from build123d import *
from OCP.BRepFilletAPI import BRepFilletAPI_MakeChamfer

# Parameters (mm, degrees)
SKETCH1_R           = 10
BOSS_EXTRUDE1_DEPTH = 28.5
BOSS_EXTRUDE2_DEPTH = 45
CUT_EXTRUDE1_DEPTH  = 30
CIRPATTERN1_COUNT   = 2
CHAMFER1_SIZE       = 50
CHAMFER1_SIZE2      = 13.397459622
FILLET3_R           = 15
CHAMFER2_SIZE       = 90
CHAMFER2_SIZE2      = 13.607292824
CUT_EXTRUDE2_DEPTH  = 138.877715566
CUT_EXTRUDE4_DEPTH  = 22.15
FILLET6_R           = 6.35


with BuildPart() as part:
    # Sketch1 → Boss-Extrude1 (new body)
    with BuildSketch(Plane.XY):
        Polygon((-9.192766332, -123.5075), (41.607233668, 123.5075), (9.192766332, 123.5075), (-41.607233668, -123.5075), align=None)
        with Locations(Location((0, 0, 0), (0, 0, 180))):
            Circle(SKETCH1_R, mode=Mode.SUBTRACT)
    extrude(amount=BOSS_EXTRUDE1_DEPTH)

    # Sketch2 → Boss-Extrude2 (add)
    with BuildSketch(Plane(origin=(0, 0, 0), x_dir=(-1, 0, 0), z_dir=(0, 0, -1))):
        Polygon((-41.607233668, 123.5075), (-38.473043437, 108.2675), (-6.0585761, 108.2675), (-9.192766332, 123.5075), align=None)
        Polygon((38.473043437, -108.2675), (6.0585761, -108.2675), (9.192766332, -123.5075), (41.607233668, -123.5075), align=None)
    extrude(amount=BOSS_EXTRUDE2_DEPTH)

    # Sketch4 → Cut-Extrude1 (cut)
    with BuildSketch(Plane(origin=(0, 123.5075, 0), x_dir=(1, 0, 0), z_dir=(0, 1, 0))):
        with BuildLine():
            ThreePointArc((20.6375, 30.433032299), (22.032403955, 27.065436254), (25.4, 25.670532299))
            Line((25.4, 25.670532299), (25.4, 30.433032299))
            Line((25.4, 30.433032299), (20.6375, 30.433032299))
        make_face()
        with BuildLine():
            Line((25.4, 30.433032299), (25.4, 25.670532299))
            ThreePointArc((25.4, 25.670532299), (28.767596045, 27.065436254), (30.1625, 30.433032299))
            Line((30.1625, 30.433032299), (25.4, 30.433032299))
        make_face()
        with BuildLine():
            Line((20.6375, 30.433032299), (25.4, 30.433032299))
            Line((25.4, 30.433032299), (25.4, 35.195532299))
            ThreePointArc((25.4, 35.195532299), (22.032403955, 33.800628344), (20.6375, 30.433032299))
        make_face()
        with BuildLine():
            Line((25.4, 35.195532299), (25.4, 30.433032299))
            Line((25.4, 30.433032299), (30.1625, 30.433032299))
            ThreePointArc((30.1625, 30.433032299), (28.767596045, 33.800628344), (25.4, 35.195532299))
        make_face()
    cut_extrude1 = extrude(amount=-CUT_EXTRUDE1_DEPTH, mode=Mode.SUBTRACT)

    # CirPattern1: Cut-Extrude1 ×2 about axis
    cirpattern1_axis = Axis((0, 0, 28.5), (0, 0, -1))
    for i in range(1, CIRPATTERN1_COUNT):
        add(cut_extrude1.rotate(cirpattern1_axis, i * 360 / CIRPATTERN1_COUNT), mode=Mode.SUBTRACT)

    # Chamfer1: one chamfer whose edges measure the first distance from different faces: ONE call of the kernel's chamfer builder (chamfer() names one face for all edges)
    chamfer1_edges_1 = [part.edges().sort_by_distance(p)[0] for p in [
        (-25.4, -123.5075, 28.5),
    ]]
    chamfer1_side_1 = [part.faces().sort_by_distance(p)[0] for p in [
        (-25.4, -123.5075, -7.566085514),
    ]]
    chamfer1_edges_2 = [part.edges().sort_by_distance(p)[0] for p in [
        (25.4, 123.5075, 28.5),
    ]]
    chamfer1_side_2 = [part.faces().sort_by_distance(p)[0] for p in [
        (25.4, 123.5075, -7.566085514),
    ]]
    chamfer1 = BRepFilletAPI_MakeChamfer(part.part.solid().wrapped)
    for e in chamfer1_edges_1:
        chamfer1.Add(CHAMFER1_SIZE, CHAMFER1_SIZE2, e.wrapped, chamfer1_side_1[0].wrapped)  # the first distance lies on this face
    for e in chamfer1_edges_2:
        chamfer1.Add(CHAMFER1_SIZE, CHAMFER1_SIZE2, e.wrapped, chamfer1_side_2[0].wrapped)  # the first distance lies on this face
    add(Compound.cast(chamfer1.Shape()), mode=Mode.REPLACE)

    # Fillet3
    fillet3_edges = [part.edges().sort_by_distance(p)[0] for p in [
        (22.265809769, 108.2675, 0),
        (-22.265809769, -108.2675, 0),
    ]]
    fillet(fillet3_edges, radius=FILLET3_R)

    # Chamfer2
    chamfer2_edges = [part.edges().sort_by_distance(p)[0] for p in [
        (-22.644738381, -110.110040378, 28.5),
        (22.644738381, 110.110040378, 28.5),
    ]]
    chamfer2_side = [part.faces().sort_by_distance(p)[0] for p in [
        (13.919836124, 0.470415947, 28.5),
    ]]
    chamfer(chamfer2_edges, length=CHAMFER2_SIZE, length2=CHAMFER2_SIZE2, reference=chamfer2_side[0])

    # Sketch10 → Cut-Extrude2 (cut, symmetric)
    with BuildSketch(Plane(origin=(0, 0, 0), x_dir=(0, 0, -1), z_dir=(1, 0, 0))):
        with BuildLine():
            Line((-28.5, 20.110040378), (-11.939027322, 98.927851264))
            ThreePointArc((-11.939027322, 98.927851264), (-4.989688501, 112.1926981), (7.875417438, 119.856804105))
            Line((7.875417438, 119.856804105), (-24.698068362, 128.387749722))
            Line((-24.698068362, 128.387749722), (-33.956814005, 23.522391457))
            Line((-33.956814005, 23.522391457), (-28.5, 20.110040378))
        make_face()
    cut_extrude2 = extrude(amount=CUT_EXTRUDE2_DEPTH, both=True, mode=Mode.SUBTRACT)

    # Mirror1: Cut-Extrude2 across plane
    add(cut_extrude2.mirror(Plane.ZX), mode=Mode.SUBTRACT)

    # Sketch11 → Cut-Extrude4 (cut)
    with BuildSketch(Plane.XY.offset(28.5)):
        Polygon((15.129215341, 26.281205366), (-4.316825144, 26.294041963), (9.314806588, 92.577851264), (28.763486991, 92.577851264), align=None)
        Polygon((-15.165993749, -26.460040378), (4.282686653, -26.460040378), (-9.314806588, -92.577851264), (-28.763486991, -92.577851264), align=None)
    extrude(amount=-CUT_EXTRUDE4_DEPTH, mode=Mode.SUBTRACT)

    # Fillet6
    fillet6_edges = [part.edges().sort_by_distance(p)[0] for p in [
        (15.129215341, 26.281205366, 16.776666244),
        (-4.316825144, 26.294041963, 16.775317649),
        (9.314806588, 92.577851264, 9.811635567),
        (28.763486991, 92.577851264, 9.811635567),
        (-28.763486991, -92.577851264, 9.811635567),
        (-9.314806588, -92.577851264, 9.811635567),
        (4.282686653, -26.460040378, 16.757878094),
        (-15.165993749, -26.460040378, 16.757878094),
    ]]
    fillet(fillet6_edges, radius=FILLET6_R)


solid = part.part
Can you work these out from the model? Positions are in its coordinate system, mm. A direction names the side the tool comes from. Round coordinates to 2 decimals unless told otherwise and drop trailing zeros. Write each loop counter-clockwise with the first axis right and the second up, starting at its lowest first coordinate (ties: lowest second). Pieces come first, ordered by that corner, then holes. Notation, with made-up numbers: M -19,0 L 11,0 A29 cw 11,35 Z; hole C -17,51 d9. An arc over 180 degrees is marked long. Use a Markdown table: item, result.
Item 1: We'd pull the mould along Y, two halves only. Please class faces 6 (the face through (-22.24, -112.038, 5.135)), 7 (the face through (1.549, 59.335, 20.258)), 8 (the face through (10.43, 91.11, 10.29)): released by +Y, released by -Y, zero draft, split by the parting line, or undercut.
Found:
| item | result |
|---|---|
| face 6 | released by -Y |
| face 7 | released by +Y |
| face 8 | undercut |
Item 2: I want a section at D-D (y = 95.5). List the corners of the cut face in (x, z) for me, and give its area (3 significant figures).
Found:
| item | result |
|---|---|
| outline | M 3.43,-0.17 L 35.85,-0.17 L 35.85,12.66 L 3.43,12.66 Z |
| area | 416 mm2 |
Item 3: I want a section at B-B (x = 0). List the corners of the cut face in (y, z) for me.
Found:
| item | result |
|---|---|
| outline | M -78.81,0 L -10,0 L -10,28.5 L -20.11,28.5 L -27.52,26.94 L -27.52,6.35 L -47.28,6.35 L -47.28,22.79 L -78.81,16.17 Z; M 10,0 L 78.81,0 L 78.81,16.17 L 47.28,22.79 L 47.28,6.35 L 27.32,6.35 L 27.32,26.98 L 20.11,28.5 L 10,28.5 Z |
Item 4: For pin 1 Ø9 at (x, y) = (9.5, 45) entering from +Z; pin 2 Ø15 at (x, z) = (30, -35) entering from -Y; pin 3 Ø10 at (x, y) = (20.5, 2) entering from -Z; pin 4 Ø2 at (y, z) = (35.5, -1.5) entering from -X, each with a flat end and sliding along its axis, tell me the tip position at first contact or that it passes through.
Found:
| item | result |
|---|---|
| pin 1 | stops at z = 6.35 |
| pin 2 | stops at y = 108.27 |
| pin 3 | stops at z = 0 |
| pin 4 | passes through |
Item 5: Which directions (+Z, -Z, +X, -X, +Y, -Y) give clear straight access to the entire face, cutting with the end or side of a thin tool? Please do faces 1 (the face through (22, 108.268, -26)), 2 (the face through (1.46, 54.38, 13.97)), 3 (the face through (15, 1, 0)), 4 (the face through (-26, -123.508, -36)), 5 (the face through (-22, -108.268, -26)).
Found:
| item | result |
|---|---|
| face 1 | -Z, +X, -X, -Y |
| face 2 | +Z |
| face 3 | -Z, +X, -X |
| face 4 | +Z, -Z, +X, -X, -Y |
| face 5 | -Z, +X, -X, +Y |
Item 6: I want a section at C-C (y = 52). List the corners of the cut face in (x, z) for me.
Found:
| item | result |
|---|---|
| outline | M -5.51,0 L 26.9,0 L 26.9,21.8 L 20.42,21.8 L 20.42,6.35 L 0.97,6.35 L 0.97,21.8 L -5.51,21.8 Z |
Item 7: I want a section at A-A (y = 0). List the corners of the cut face in (x, z) for me.
Found:
| item | result |
|---|---|
| outline | M -16.21,0 L -10,0 L -10,28.5 L -16.21,28.5 Z; M 10,0 L 16.21,0 L 16.21,28.5 L 10,28.5 Z |
Item 8: If I drill on line 1 along Z through (x, y) = (-8.5, -79.5); line 2 along Y through (x, z) = (-34, -29.5); line 3 along X through (y, z) = (-71, 8.5), over which ranges is the centre line in solid material (lowest first)? Write a range as [from, to].
Found:
| item | result |
|---|---|
| line 1 | z = [0, 6.35] |
| line 2 | y = [-123.51, -108.27] |
| line 3 | x = [-30.81, -24.33], [-4.88, 1.61] |
